from build123d import *

# Parameters (mm, degrees)
SKETCH_R     = 12
SKETCH_R_2   = 21
SKETCH_R_3   = 19.584537
SKETCH_R_4   = 3.467704
PAD_DEPTH    = 30
PAD001_DEPTH = 30


with BuildPart() as part:
    # Sketch → Pad (new body)
    with BuildSketch(Plane.XY):
        with BuildLine():
            Line((-35.584206, -63.111127), (44.415794, -63.111127))
            ThreePointArc((44.415794, -63.111127), (77.13309, -49.55918), (90.685038, -16.841884))
            Line((90.685038, -16.841884), (90.685038, 63.158116))
            ThreePointArc((90.685038, 63.158116), (77.13309, 95.875412), (44.415794, 109.427359))
            Line((44.415794, 109.427359), (-35.584206, 109.427359))
            ThreePointArc((-35.584206, 109.427359), (-68.301501, 95.875412), (-81.853449, 63.158116))
            Line((-81.853449, 63.158116), (-81.853449, -16.841884))
            ThreePointArc((-81.853449, -16.841884), (-68.301501, -49.55918), (-35.584206, -63.111127))
        make_face()
        with Locations((4.306361, 24.767706)):
            Circle(SKETCH_R, mode=Mode.SUBTRACT)
        with Locations((-50.106209, -31.898642)):
            Circle(SKETCH_R_2, mode=Mode.SUBTRACT)
        with Locations((59.362869, 78.858307)):
            Circle(SKETCH_R_3, mode=Mode.SUBTRACT)
        with Locations((-75.219696, 34.748711)):
            Circle(SKETCH_R_4, mode=Mode.SUBTRACT)
        with Locations((-64.916733, 34.748711)):
            Circle(SKETCH_R_4, mode=Mode.SUBTRACT)
        with Locations((-54.613762, 34.748711)):
            Circle(SKETCH_R_4, mode=Mode.SUBTRACT)
        with Locations((-44.954719, 34.748711)):
            Circle(SKETCH_R_4, mode=Mode.SUBTRACT)
        with Locations((-34.651756, 34.748711)):
            Circle(SKETCH_R_4, mode=Mode.SUBTRACT)
        with Locations((-24.348785, 34.748711)):
            Circle(SKETCH_R_4, mode=Mode.SUBTRACT)
        with Locations((-75.219696, 25.089674)):
            Circle(SKETCH_R_4, mode=Mode.SUBTRACT)
        with Locations((-64.916733, 25.089674)):
            Circle(SKETCH_R_4, mode=Mode.SUBTRACT)
        with Locations((-54.613762, 25.089674)):
            Circle(SKETCH_R_4, mode=Mode.SUBTRACT)
        with Locations((-44.954719, 25.089674)):
            Circle(SKETCH_R_4, mode=Mode.SUBTRACT)
        with Locations((-34.651756, 25.089674)):
            Circle(SKETCH_R_4, mode=Mode.SUBTRACT)
        with Locations((-24.348785, 25.089674)):
            Circle(SKETCH_R_4, mode=Mode.SUBTRACT)
        with Locations((34.249382, 35.392641)):
            Circle(SKETCH_R_4, mode=Mode.SUBTRACT)
        with Locations((44.552345, 35.392641)):
            Circle(SKETCH_R_4, mode=Mode.SUBTRACT)
        with Locations((54.855316, 35.392641)):
            Circle(SKETCH_R_4, mode=Mode.SUBTRACT)
        with Locations((64.514359, 35.392641)):
            Circle(SKETCH_R_4, mode=Mode.SUBTRACT)
        with Locations((74.817322, 35.392641)):
            Circle(SKETCH_R_4, mode=Mode.SUBTRACT)
        with Locations((85.120293, 35.392641)):
            Circle(SKETCH_R_4, mode=Mode.SUBTRACT)
        with Locations((34.249382, 25.733604)):
            Circle(SKETCH_R_4, mode=Mode.SUBTRACT)
        with Locations((44.552345, 25.733604)):
            Circle(SKETCH_R_4, mode=Mode.SUBTRACT)
        with Locations((54.855316, 25.733604)):
            Circle(SKETCH_R_4, mode=Mode.SUBTRACT)
        with Locations((64.514359, 25.733604)):
            Circle(SKETCH_R_4, mode=Mode.SUBTRACT)
        with Locations((74.817322, 25.733604)):
            Circle(SKETCH_R_4, mode=Mode.SUBTRACT)
        with Locations((85.120293, 25.733604)):
            Circle(SKETCH_R_4, mode=Mode.SUBTRACT)
    extrude(amount=PAD_DEPTH)

    # Sketch → Pad001 (join)
    with BuildSketch(Plane.XY):
        with BuildLine():
            Line((-35.584206, -63.111127), (44.415794, -63.111127))
            ThreePointArc((44.415794, -63.111127), (77.13309, -49.55918), (90.685038, -16.841884))
            Line((90.685038, -16.841884), (90.685038, 63.158116))
            ThreePointArc((90.685038, 63.158116), (77.13309, 95.875412), (44.415794, 109.427359))
            Line((44.415794, 109.427359), (-35.584206, 109.427359))
            ThreePointArc((-35.584206, 109.427359), (-68.301501, 95.875412), (-81.853449, 63.158116))
            Line((-81.853449, 63.158116), (-81.853449, -16.841884))
            ThreePointArc((-81.853449, -16.841884), (-68.301501, -49.55918), (-35.584206, -63.111127))
        make_face()
        with Locations((4.306361, 24.767706)):
            Circle(SKETCH_R, mode=Mode.SUBTRACT)
        with Locations((-50.106209, -31.898642)):
            Circle(SKETCH_R_2, mode=Mode.SUBTRACT)
        with Locations((59.362869, 78.858307)):
            Circle(SKETCH_R_3, mode=Mode.SUBTRACT)
        with Locations((-75.219696, 34.748711)):
            Circle(SKETCH_R_4, mode=Mode.SUBTRACT)
        with Locations((-64.916733, 34.748711)):
            Circle(SKETCH_R_4, mode=Mode.SUBTRACT)
        with Locations((-54.613762, 34.748711)):
            Circle(SKETCH_R_4, mode=Mode.SUBTRACT)
        with Locations((-44.954719, 34.748711)):
            Circle(SKETCH_R_4, mode=Mode.SUBTRACT)
        with Locations((-34.651756, 34.748711)):
            Circle(SKETCH_R_4, mode=Mode.SUBTRACT)
        with Locations((-24.348785, 34.748711)):
            Circle(SKETCH_R_4, mode=Mode.SUBTRACT)
        with Locations((-75.219696, 25.089674)):
            Circle(SKETCH_R_4, mode=Mode.SUBTRACT)
        with Locations((-64.916733, 25.089674)):
            Circle(SKETCH_R_4, mode=Mode.SUBTRACT)
        with Locations((-54.613762, 25.089674)):
            Circle(SKETCH_R_4, mode=Mode.SUBTRACT)
        with Locations((-44.954719, 25.089674)):
            Circle(SKETCH_R_4, mode=Mode.SUBTRACT)
        with Locations((-34.651756, 25.089674)):
            Circle(SKETCH_R_4, mode=Mode.SUBTRACT)
        with Locations((-24.348785, 25.089674)):
            Circle(SKETCH_R_4, mode=Mode.SUBTRACT)
        with Locations((34.249382, 35.392641)):
            Circle(SKETCH_R_4, mode=Mode.SUBTRACT)
        with Locations((44.552345, 35.392641)):
            Circle(SKETCH_R_4, mode=Mode.SUBTRACT)
        with Locations((54.855316, 35.392641)):
            Circle(SKETCH_R_4, mode=Mode.SUBTRACT)
        with Locations((64.514359, 35.392641)):
            Circle(SKETCH_R_4, mode=Mode.SUBTRACT)
        with Locations((74.817322, 35.392641)):
            Circle(SKETCH_R_4, mode=Mode.SUBTRACT)
        with Locations((85.120293, 35.392641)):
            Circle(SKETCH_R_4, mode=Mode.SUBTRACT)
        with Locations((34.249382, 25.733604)):
            Circle(SKETCH_R_4, mode=Mode.SUBTRACT)
        with Locations((44.552345, 25.733604)):
            Circle(SKETCH_R_4, mode=Mode.SUBTRACT)
        with Locations((54.855316, 25.733604)):
            Circle(SKETCH_R_4, mode=Mode.SUBTRACT)
        with Locations((64.514359, 25.733604)):
            Circle(SKETCH_R_4, mode=Mode.SUBTRACT)
        with Locations((74.817322, 25.733604)):
            Circle(SKETCH_R_4, mode=Mode.SUBTRACT)
        with Locations((85.120293, 25.733604)):
            Circle(SKETCH_R_4, mode=Mode.SUBTRACT)
    extrude(amount=PAD001_DEPTH)


solid = part.part
CAD build for the part. Positions are in the model's coordinates, mm. Round coordinates to 2 decimals unless told otherwise and drop trailing zeros. Write each loop counter-clockwise with the first axis right and the second up, starting at its lowest first coordinate (ties: lowest second). Pieces come first, ordered by that corner, then holes. Notation, with made-up numbers: M 81.5,-13 L 138.5,-13 A7 cw 138.5,-8 Z; hole C -25.75,79 d5. An arc over 180 degrees is marked long. Put each result on its own line as item: value. Start each with the question number.
1) Saw through at B-B, the plane x = -5.5. Write the cut outline in (y, z).
2) Saw through at D-D, the plane z = 5. Count the separate pieces of the cut face and the enclosed holes in it, and give its area (3 significant figures).
3) Saw through at C-C, the plane x = 34. Write the cut outline in (y, z).
4) Pull direction Y, two halves, no side cores. Call faces 1 (the flat face through (22, 24, 0)), 2 (the cylindrical face through (1.705, 13.053, 14.79)), 3 (the cylindrical face through (76.77, -49.92, 14.79)): pulls with the +Y half, pulls with the -Y half, needs draft (parallel to the pull), parting line crosses it, or undercut.
5) Drill centre lines: probe 1 along Y at (x, z) = (-34, 18.5); probe 2 along Y at (x, z) = (55, 16); probe 3 along Y at (x, z) = (-73.5, 8). Where is each one in solid material? Low to high. Write a range as [from, to].
6) Saw through at A-A, the plane y = -23.5. Write the cut outline in (x, z).
7) Pin check, flat tips, straight feed: pin 1 Ø5 at (x, z) = (-59.5, 20.5) entering from +Y; pin 2 Ø6 at (x, y) = (-64.92, 25.09) entering from -Z; pin 3 Ø3 at (x, z) = (66.5, 22.5) entering from -Y; pin 4 Ø1.5 at (x, z) = (68, 24.5) entering from +Y. Stop position of each tip, or through.
Resolved:
1. outline: M -63.11,0 L 17.85,0 L 17.85,30 L -63.11,30 Z; M 31.68,0 L 109.43,0 L 109.43,30 L 31.68,30 Z
2. separate pieces: 1
2. enclosed holes: 27
2. area: 24,000 mm²
3. outline: M -63.11,0 L 22.27,0 L 22.27,30 L -63.11,30 Z; M 29.19,0 L 31.93,0 L 31.93,30 L 29.19,30 Z; M 38.85,0 L 109.43,0 L 109.43,30 L 38.85,30 Z
4. face 1: needs draft
4. face 2: undercut
4. face 3: pulls with the -Y half
5. probe 1: [-63.11, -45.37], [-18.42, 21.68], [28.5, 31.34], [38.15, 109.43]
5. probe 2: [-61.88, 22.27], [29.2, 31.93], [38.86, 59.77], [97.95, 108.2]
5. probe 3: [-43.36, 22.08], [28.1, 31.74], [37.76, 89.68]
6. outline: M -81.37,0 L -69.35,0 L -69.35,30 L -81.37,30 Z; M -30.86,0 L 90.2,0 L 90.2,30 L -30.86,30 Z
7. pin 1: y = 104.17
7. pin 2: through
7. pin 3: y = -58.28
7. pin 4: y = 103.4
